```python
from build123d import *

# Parameters (mm, degrees)
BOX005_W     = 14
BOX005_H     = 89
BOX005_DEPTH = 10
BOX004_W     = 46
BOX004_H     = 130
BOX004_DEPTH = 23
BOX003_W     = 66
BOX003_H     = 87
BOX003_DEPTH = 10
BOX002_W     = 140
BOX002_H     = 89
BOX002_DEPTH = 29
BOX001_W     = 75
BOX001_H     = 150
BOX001_DEPTH = 22
BOX_W        = 160
BOX_H        = 95
BOX_DEPTH    = 35


with BuildPart() as cubo005:
    # Box005 → Box005 (new body)
    with BuildSketch(Plane(origin=(132, 3, 22), x_dir=(1, 0, 0), z_dir=(0, 0, 1))):
        with Locations((7, 44.5)):
            Rectangle(BOX005_W, BOX005_H)
    extrude(amount=BOX005_DEPTH)


with BuildPart() as cubo004:
    # Box004 → Box004 (new body)
    with BuildSketch(Plane(origin=(100, -4, 6), x_dir=(1, 0, 0), z_dir=(0, 0, 1))):
        with Locations((23, 65)):
            Rectangle(BOX004_W, BOX004_H)
    extrude(amount=BOX004_DEPTH)


with BuildPart() as cubo003:
    # Box003 → Box003 (new body)
    with BuildSketch(Plane(origin=(71, 4, 0), x_dir=(1, 0, 0), z_dir=(0, 0, 1))):
        with Locations((33, 43.5)):
            Rectangle(BOX003_W, BOX003_H)
    extrude(amount=BOX003_DEPTH)


with BuildPart() as esfera:
    # Sphere → Sphere (revolve)
    with BuildSketch(Plane(origin=(152, 45, 17), x_dir=(1, 0, 0), z_dir=(0, -1, 0))):
        with BuildLine():
            ThreePointArc((0, -16), (16, 0), (0, 16))
            Line((0, 16), (0, -16))
        make_face()
    revolve(axis=Axis((152, 45, 17), (0, 0, 1)))


with BuildPart() as cubo002:
    # Box002 → Box002 (new body)
    with BuildSketch(Plane(origin=(0, 3, 3), x_dir=(1, 0, 0), z_dir=(0, 0, 1))):
        with Locations((70, 44.5)):
            Rectangle(BOX002_W, BOX002_H)
    extrude(amount=BOX002_DEPTH)


with BuildPart() as cubo001:
    # Box001 → Box001 (new body)
    with BuildSketch(Plane(origin=(9, 0, 7), x_dir=(1, 0, 0), z_dir=(0, 0, 1))):
        with Locations((37.5, 75)):
            Rectangle(BOX001_W, BOX001_H)
    extrude(amount=BOX001_DEPTH)


with BuildPart() as cut005:
    # Box → Box (new body)
    with BuildSketch(Plane.XY):
        with Locations((80, 47.5)):
            Rectangle(BOX_W, BOX_H)
    extrude(amount=BOX_DEPTH)

    # Cut: cut Cubo001
    add(cubo001.part, mode=Mode.SUBTRACT)

    # Cut001: cut Cubo002
    add(cubo002.part, mode=Mode.SUBTRACT)

    # Cut002: cut Esfera
    add(esfera.part, mode=Mode.SUBTRACT)

    # Cut003: cut Cubo003
    add(cubo003.part, mode=Mode.SUBTRACT)

    # Cut004: cut Cubo004
    add(cubo004.part, mode=Mode.SUBTRACT)

    # Cut005: cut Cubo005
    add(cubo005.part, mode=Mode.SUBTRACT)


solid = cut005.part
```
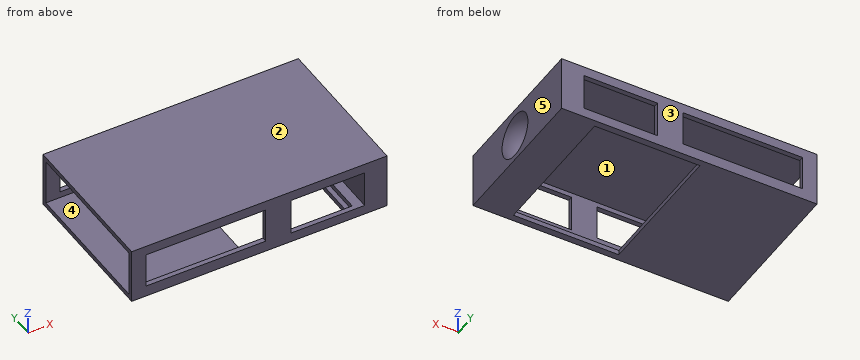
Input: part model. Units: mm. Frame: model coordinates. Face numbers are marked on the shaded views. A direction names the side the tool comes from. Round coordinates to 2 decimals unless told otherwise and drop trailing zeros. Write each loop counter-clockwise with the first axis right and the second up, starting at its lowest first coordinate (ties: lowest second). Pieces come first, ordered by that corner, then holes. Notation, with made-up numbers: M 87,89 L 107,89 A9 ccw 107,105 Z; hole C 5,-30 d4. An arc over 180 degrees is marked long. Write each question's results on one line, items separated by ' | '.
Q1. Section query B-B (x = 16). Return loops of the section in (y, z), and give its area (3 significant figures).
Results:
outline: M 0,0 L 95,0 L 95,7 L 92,7 L 92,3 L 3,3 L 3,7 L 0,7 Z; M 0,29 L 3,29 L 3,32 L 92,32 L 92,29 L 95,29 L 95,35 L 0,35 Z | area: 612 mm^2
Q2. Pin query (flat end, axial travel): P1, Ø1.5, axis at y = 55.5, z = 4, coming from the -X side. Return the tip coordinate at first contact, or that it passes through.
Results:
P1: stops at x = 140
Q3. Line query: line 1 along Z through (x, y) = (36, 11); line 2 along Y through (x, z) = (41.5, 30); line 3 along Z through (x, y) = (99, 33). Output: solid intervals per line, ascending.
Results:
line 1: z = 0 to 3, 32 to 35 | line 2: y = 0 to 3, 92 to 95 | line 3: z = 32 to 35
Q4. Section query A-A (y = 19). Return loops of the section in (x, z).
Results:
outline: M 0,0 L 71,0 L 71,3 L 0,3 Z; M 0,32 L 146,32 L 146,6 L 140,6 L 140,3 L 137,3 L 137,0 L 160,0 L 160,35 L 0,35 Z
Q5. Section query C-C (x = 121). Return loops of the section in (y, z).
Results:
outline: M 0,0 L 4,0 L 4,3 L 3,3 L 3,6 L 0,6 Z; M 0,29 L 3,29 L 3,32 L 92,32 L 92,29 L 95,29 L 95,35 L 0,35 Z; M 91,0 L 95,0 L 95,6 L 92,6 L 92,3 L 91,3 Z
Q6. Section query D-D (z = 11.5). Return loops of the section in (x, y), and give its area (3 significant figures).
Results:
outline: M 0,0 L 9,0 L 9,3 L 0,3 Z; M 0,92 L 9,92 L 9,95 L 0,95 Z; M 84,0 L 100,0 L 100,3 L 84,3 Z; M 84,92 L 100,92 L 100,95 L 84,95 Z; M 146,0 L 160,0 L 160,32.28 A15.02 cw 146,31.23 Z; M 146,58.77 A15.02 cw 160,57.72 L 160,95 L 146,95 Z | area: 1,080 mm^2
Q7. Access query for the marked faces 4 and 5. Directions: +Z, -Z, +X, -X, +Y, -Y. A direction counts if a zero-diameter tool reaches every point of the face in a straight line with its end or side. Return the directions, or none.
Results:
face 4: -X | face 5: +Z, -Z, +X, +Y, -Y
Q8. Draft query along Y for the marked faces 1, 2 and 3. Return one class per face: released by +Y, released by -Y, zero draft, split by the parting line, or undercut.
Results:
face 1: undercut | face 2: zero draft | face 3: released by +Y
